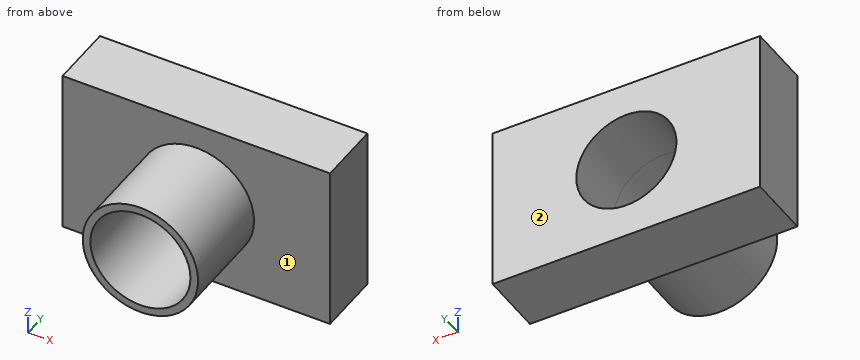
```python
from build123d import *

# Parameters (mm, degrees)
F0_W      = 127.534748
F0_H      = 79.408422
F1_DEPTH  = 15.24
F2_R      = 27.530043
F2_R_2    = 23.859261
F3_DEPTH  = 45.72
F3_FACE_R = 23.859261
F4_DEPTH  = 46.99


with BuildPart() as f1:
    # F0 (on Front) → F1 (new body, symmetric)
    with BuildSketch(Plane.XZ):
        Rectangle(F0_W, F0_H)
    extrude(amount=F1_DEPTH, both=True)

    # F2 (on face) → F3 (join)
    with BuildSketch(Plane.XZ.offset(15.24)):
        Circle(F2_R)
        Circle(F2_R_2, mode=Mode.SUBTRACT)
    extrude(amount=F3_DEPTH)

    # F3_face (on face) → F4 (cut)
    with BuildSketch(Plane.XZ.offset(15.24)):
        Circle(F3_FACE_R)
    extrude(amount=-F4_DEPTH, mode=Mode.SUBTRACT)


solid = f1.part
```
Here's how the part is built. I have some questions about the finished solid (model axes, mm). Face numbers are marked on the shaded views. A direction names the side the tool comes from. Coordinates: 2 decimals unless noted, no trailing zeros. Write each loop counter-clockwise with the first axis right and the second up, starting at its lowest first coordinate (ties: lowest second). Pieces come first, ordered by that corner, then holes. Notation, with made-up numbers: M 16,-15 L 69,-15 A31 cw 69,16 Z; hole C 71.5,-10.75 d9. An arc over 180 degrees is marked long. Answer as CSV lines item,"result". Start each with the question number.
Q1. Will these pins go through, and if not, where does the flat tip stop? pin 1 Ø12 at (x, z) = (-34.5, 28.5) entering from -Y; pin 2 Ø8 at (y, z) = (-19.5, -5.5) entering from +X; pin 3 Ø1.5 at (x, y) = (-25, -51.5) entering from -Z.
Q2. Suppose I cut it at A-A, the plane z = 0. List the corners of the cut face in (x, y) for me.
Q3. Suppose I cut it at B-B, the plane x = 0. List the corners of the cut face in (y, z) for me.
Q4. Suppose I cut it at C-C, the plane y = -9.5. List the corners of the cut face in (x, z) for me.
Q5. For the marked faces 1 and 2, which set-ups out of +Z, -Z, +X, -X, +Y, -Y let a thin tool reach every point of the face, with its end or its side?
Q6. I need wall thicknesses on probe 1 along Z at (x, y) = (0, 0); probe 2 along Z at (x, y) = (0, -28.5); probe 3 along Y at (x, z) = (-32, -31.5). Which ranges of each line are inside material? Lowest first, please. Write a range as [from, to].
Q7. Suppose I cut it at D-D, the plane x = -30. List the corners of the cut face in (y, z) for me, then the cut area to 3 significant figures.
Entries:
1,pin 1,"stops at y = -15.24"
1,pin 2,"stops at x = 27.49"
1,pin 3,"stops at z = -13.03"
2,outline,"M -63.77,-15.24 L -27.53,-15.24 L -27.53,-60.96 L -23.86,-60.96 L -23.86,15.24 L -63.77,15.24 Z; M 23.86,-60.96 L 27.53,-60.96 L 27.53,-15.24 L 63.77,-15.24 L 63.77,15.24 L 23.86,15.24 Z"
3,outline,"M -60.96,-27.53 L -15.24,-27.53 L -15.24,-39.7 L 15.24,-39.7 L 15.24,-23.86 L -60.96,-23.86 Z; M -60.96,23.86 L 15.24,23.86 L 15.24,39.7 L -15.24,39.7 L -15.24,27.53 L -60.96,27.53 Z"
4,outline,"M -63.77,-39.7 L 63.77,-39.7 L 63.77,39.7 L -63.77,39.7 Z; hole C 0,0 d47.72"
5,face 1,"-Y"
5,face 2,"+Z, -Z, +X, -X, +Y"
6,probe 1,"z = [-39.7, -23.86], [23.86, 39.7]"
6,probe 2,"z = [-27.53, -23.86], [23.86, 27.53]"
6,probe 3,"y = [-15.24, 15.24]"
7,outline,"M -15.24,-39.7 L 15.24,-39.7 L 15.24,39.7 L -15.24,39.7 Z"
7,area,"2,420 mm²"
